Autodesk Inventor part; units mm, degrees
ref_plane "YZ Plane" through (0, 0, 0) normal (1, 0, 0) x (0, 1, 0)
ref_plane "XZ Plane" through (0, 0, 0) normal (0, 1, 0) x (-1, 0, 0)
ref_plane "XY Plane" through (0, 0, 0) normal (0, 0, 1) x (1, 0, 0)
sketch "Sketch1" plane through (0, 0, 0) normal (0, 1, 0) x (-1, 0, 0)
  circle A0 centre (0, 0) radius 74.3
  circle A1 centre (0, 0) radius 62.3
  line L0 (62.3, 0) -> (74.3, 0) construction
  point P0 (68.3, 0)
  point P1 (0, 68.3)
  point P2 (-68.3, 0)
  point P3 (0, -68.3)
  dimension "d0" = 148.6
  dimension "d1" = 12
  dimension "d4" = 360
extrude "Extrusion1" add sketch "Sketch1" along normal blind 10
hole "Hole1" at (-68.3, 0, 0) at (0, 0, 68.3) at (68.3, 0, 0) at (0, 0, -68.3) direction (0, 1, 0) diameter 5 end through all countersink diameter 10.3886 countersink angle 90
properties part number "OR"
Geometry check sheet. Reference: the model listing, model coordinates, mm. Round coordinates to 2 decimals unless told otherwise and drop trailing zeros. Order: outer loops, then holes, each group sorted by start corner. A loop starts at its lowest first (then second) coordinate and runs counter-clockwise, first axis right, second up. Notation, with made-up numbers: (-18.75, 42) - (34.25, 42) arc R22 ccw to (34.25, 49) - close; hole circle Ø3 at (70.5, -25). An arc over 180 degrees is marked (long way). Use a Markdown table: item, result. Add a question column.
(1) Material ranges on line 1 along Z through (x, y) = (0, 8); line 2 along X through (y, z) = (4.75, -13); line 3 along X through (y, z) = (0.5, -52), recorded low to high. Write a range as [from, to].
(2) Sectioned sample at A-A, the plane y = 6. Enter the section's corners in (x, z).
(3) Release check for a two-part mould opening along Z. For faces 1 (the flat face through (16.9, 10, -60.2)), 2 (the cylindrical face through (70.74, 6.4, 0.54)), 3 (the cylindrical face through (9.67, 4.93, -73.67)), 4 (the conical face through (-1, 2.5, -70.8)) record: pulls with the +Z half, pulls with the -Z half, needs draft (parallel to the pull), parting line crosses it, or undercut.
(4) Sectioned sample at B-B, the plane z = 50. Enter the section's corners in (x, y).
(5) Sectioned sample at D-D, the plane z = -31. Enter the section's corners in (x, y), and give its area (3 significant figures).
(6) Depth check by flat-ended pin: pin 1 (1 mm diameter, centred on y = 6.5, z = -49, fed in from -X); pin 2 (3 mm diameter, centred on y = 4.5, z = 47, fed in from -X); pin 3 (1 mm diameter, centred on y = 3, z = 1, fed in from -X). Enter the tip coordinate at first touch or a pass-through.
(7) Sectioned sample at C-C, the plane x = -68.3. Enter the section's corners in (y, z), and give its area (3 significant figures).
Answers below:
| question | item | result |
|---|---|---|
| 1 | line 1 | [-74.3, -70.8], [-65.8, -62.3], [62.3, 65.8], [70.8, 74.3] |
| 1 | line 2 | [-73.15, -60.93], [60.93, 73.15] |
| 1 | line 3 | [-53.07, -34.31], [34.31, 53.07] |
| 2 | outline | circle Ø148.6 at (0, 0); hole circle Ø5 at (-68.3, 0); hole circle Ø124.6 at (0, 0); hole circle Ø5 at (0, -68.3); hole circle Ø5 at (0, 68.3); hole circle Ø5 at (68.3, 0) |
| 3 | face 1 | needs draft |
| 3 | face 2 | undercut |
| 3 | face 3 | parting line crosses it |
| 3 | face 4 | undercut |
| 4 | outline | (-54.96, 0) - (-37.17, 0) - (-37.17, 10) - (-54.96, 10) - close; (37.17, 0) - (54.96, 0) - (54.96, 10) - (37.17, 10) - close |
| 5 | outline | (-67.52, 0) - (-54.04, 0) - (-54.04, 10) - (-67.52, 10) - close; (54.04, 0) - (67.52, 0) - (67.52, 10) - (54.04, 10) - close |
| 5 | area | 270 mm² |
| 6 | pin 1 | x = -56.29 |
| 6 | pin 2 | x = -58.74 |
| 6 | pin 3 | x = -74.3 |
| 7 | outline | (0, -29.25) - (10, -29.25) - (10, -2.5) - (2.69, -2.5) - (0, -5.19) - close; (0, 5.19) - (2.69, 2.5) - (10, 2.5) - (10, 29.25) - (0, 29.25) - close |
| 7 | area | 528 mm² |
